Read the model definition and answer for the solid it produces. Units are mm, in the model's axes. A direction names the side the tool comes from. Coordinates: 2 decimals unless noted, no trailing zeros. Loops run counter-clockwise (first coordinate to the right, second up) from the corner with the lowest first, then second, coordinate; pieces in that order, holes last.
Q1. Section D-D (y = 54.25) is taken. Give the vertices of the cut face in (x, z).
Q2. Which of the six approach directions +Z, -Z, +X, -X, +Y, -Y give full straight-line access (tool end or side, diameter ignored) to faces 4 (the face through (-32, 65.5, 38)), 5 (the face through (-32, 57, 44)), 6 (the face through (-28, 59, 39))?
Q3. Straight lines are drawn through the part: line 1 (X direction, y = 56.5, z = 38); line 2 (Y direction, x = -33.5, z = 40); line 3 (Y direction, x = -33, z = 44.75). For each, find the intervals that lie inside material, in ascending order.
Q4. The mould has two halves that part along X. Classify faces 1 (the face through (-33, 70, 39)), 2 (the face through (-32, 63, 44)), 3 (the face through (-37, 59, 39)): pulls with the +X half, pulls with the -X half, needs draft (parallel to the pull), parting line crosses it, or undercut.
Q5. Section A-A (y = 62.75) is taken. Give the vertices of the cut face in (x, z).
Q6. Section B-B (x = -35.5) is taken. Give the vertices of the cut face in (y, z).
Q7. A flat-ended cylindrical pin translates along its axis: P1, Ø2, axis at x = -34, y = 64, coming from the -Z side. Find the tip coordinate at first contact, or state that the pin passes through.
Q8. Section C-C (z = 44) is taken. Give the vertices of the cut face in (x, y).
from build123d import *

# Parameters (mm, degrees)
BOX049_W                     = 6
BOX049_H                     = 7
BOX049_DEPTH                 = 8
BOX048_W                     = 7
BOX048_H                     = 12
BOX048_DEPTH                 = 10
CHAMFER001_SIZE              = 1
CHAMFER001_PLACEMENT_ANGLE   = 90
FUSION002028_PLACEMENT_ANGLE = 90
BOX047_W                     = 9
BOX047_H                     = 21
BOX047_DEPTH                 = 11


with BuildPart() as cubo049:
    # Box049 → Box049 (new body)
    with BuildSketch(Plane(origin=(-9.5, -15, 2.5), x_dir=(1, 0, 0), z_dir=(0, 0, 1))):
        with Locations((3, 3.5)):
            Rectangle(BOX049_W, BOX049_H)
    extrude(amount=BOX049_DEPTH)


with BuildPart() as fusion002028:
    # Box048 → Box048 (new body)
    with BuildSketch(Plane(origin=(-13, -7, 7.5), x_dir=(1, 0, 0), z_dir=(0, 0, -1))):
        with Locations((3.5, 6)):
            Rectangle(BOX048_W, BOX048_H)
    extrude(amount=BOX048_DEPTH)

    # Chamfer001
    chamfer001_edges = [fusion002028.edges().sort_by_distance(p)[0] for p in [
        (-13, -13, -2.5),
    ]]
    chamfer(chamfer001_edges, length=CHAMFER001_SIZE)


with BuildPart() as fusion002028_1:
    # Chamfer001 placement: moved
    add(fusion002028.part.moved(Location((-20, -2, 0.5))).rotate(Axis((-20, -2, 0.5), (0, 0, 1)), CHAMFER001_PLACEMENT_ANGLE))

    # Fusion002028: union Cubo049
    add(cubo049.part)


with BuildPart() as fusion002028_2:
    # Fusion002028 placement: moved
    add(fusion002028_1.part.moved(Location((-44, 66.5, 34.8))).rotate(Axis((-44, 66.5, 34.8), (0, 0, 1)), FUSION002028_PLACEMENT_ANGLE))


with BuildPart() as cut072:
    # Box047 → Box047 (new body)
    with BuildSketch(Plane(origin=(-37, 49, 34), x_dir=(1, 0, 0), z_dir=(0, 0, 1))):
        with Locations((4.5, 10.5)):
            Rectangle(BOX047_W, BOX047_H)
    extrude(amount=BOX047_DEPTH)

    # Cut072: cut Fusion002028
    add(fusion002028_2.part, mode=Mode.SUBTRACT)


solid = cut072.part
Numbers:
1. outline: (-37, 34) - (-36, 34) - (-36, 42.8) - (-29, 42.8) - (-29, 34) - (-28, 34) - (-28, 45) - (-37, 45) - close
2. face 4: -Z
2. face 5: +Z, -Z
2. face 6: +Z, -Z, +X, +Y, -Y
3. line 1: x = -37 to -36, -29 to -28
3. line 2: y = 49 to 53.5, 65.5 to 70
3. line 3: y = 49 to 57, 63 to 70
4. face 1: needs draft
4. face 2: undercut
4. face 3: pulls with the -X half
5. outline: (-37, 34) - (-36, 34) - (-36, 45) - (-37, 45) - close; (-29, 34) - (-28, 34) - (-28, 45) - (-29, 45) - close
6. outline: (49, 34) - (53.5, 34) - (53.5, 42.8) - (57, 42.8) - (57, 45) - (49, 45) - close; (63, 42.8) - (65.5, 42.8) - (65.5, 34) - (70, 34) - (70, 45) - (63, 45) - close
7. P1: stops at z = 42.8
8. outline: (-37, 49) - (-28, 49) - (-28, 70) - (-37, 70) - close; hole (-36, 57) - (-29, 57) - (-29, 63) - (-36, 63) - close
